```python
from build123d import *

# Parameters (mm, degrees)
F2_W     = 3.429
F2_H     = 3.429
F3_DEPTH = 25.4
F4_R     = 1.26999
F5_R     = 1.26999


# Not quite as in the source:
# - a fillet or chamfer is up to 0.001 mm smaller than in the source, because OpenCascade refuses the exact size


with BuildPart() as f1:
    # F0 (on Front) → F1 (revolve)
    with BuildSketch(Plane.XZ):
        Polygon((-1.27, 0), (0, 0), (4.445, 0), (4.445, 10.16), (0, 10.16), (-1.27, 10.16), (-1.27, 8.89), (0, 8.89), (0, 1.27), (-1.27, 1.27), align=None)
    revolve(axis=Axis((4.445, 0, 5.08), (0, 0, -1)))

    # F2 (on face) → F3 (cut)
    with BuildSketch(Plane(origin=(0, 0, 0), x_dir=(1, 0, 0), z_dir=(0, 0, -1))):
        with Locations((4.445, 0)):
            Rectangle(F2_W, F2_H)
    extrude(amount=-F3_DEPTH, mode=Mode.SUBTRACT)

    # F4 (radius 1.27 in the source; OpenCascade refuses exactly that, so slightly less here)
    f4_edges = [f1.edges().sort_by_distance(p)[0] for p in [
        (10.16, 0, 0),
    ]]
    fillet(f4_edges, radius=F4_R)

    # F5 (radius 1.27 in the source; OpenCascade refuses exactly that, so slightly less here)
    f5_edges = [f1.edges().sort_by_distance(p)[0] for p in [
        (10.16, 0, 10.16),
    ]]
    fillet(f5_edges, radius=F5_R)


solid = f1.part
```
Work out the finished part from the listing and answer in its coordinate system (mm). A direction names the side the tool comes from. Give positions to 0.01 mm unless a question says otherwise; leave off trailing zeros. Order: outer loops, then holes, each group sorted by start corner. A loop starts at its lowest first (then second) coordinate and runs counter-clockwise, first axis right, second up. Notation, with made-up numbers: (-27, -11) -> (-18, -11) arc R24 cw to (-18, 18) -> close; hole circle Ø3 at (8, 54). An arc over 180 degrees is marked (long way). Answer as CSV lines item,"result". Start each with the question number.
(1) For a pull along Z with two mould halves and no side action, classify faces 1 (the flat face through (8, -3, 8.89)), 2 (the flat face through (6.4, 0.1, 10.16)), 3 (the flat face through (4, -1.714, 5)) as released by +Z, released by -Z, zero draft, split by the parting line, or undercut.
(2) Each of these flat-tipped pins is pushed along its axis until it touches: pin 1 Ø1.7 at (y, z) = (0, 6.5) entering from +X; pin 2 Ø1.7 at (y, z) = (-0.5, 7) entering from -X; pin 3 Ø1 at (x, z) = (5, 2.5) entering from +Y. Where does it stop, or does it pass through?
(3) Section C-C, the plane z = 9.25 is taken. Write down the section's boundary in (x, y) (1 decimal).
(4) Consider line 1 along Y through (x, z) = (4.25, 7.75); line 2 along X through (y, z) = (0.5, 5); line 3 along Y through (x, z) = (4.25, 9). Determine where each line is inside the solid, lowest interval first.
(5) Which of the six approach directions +Z, -Z, +X, -X, +Y, -Y give full straight-line access (tool end or side, diameter ignored) to faces 4 (the cylindrical face through (5.41, -4.34, 5.03)), 5 (the flat face through (2.5, 0.1, 0)), 6 (the flat face through (6.16, 0, 5))?
(6) Section B-B, the plane z = 2.5 is taken. Write down the section's boundary in (x, y) (1 decimal), plus the area to 3 significant figures.
Entries:
1,face 1,"undercut"
1,face 2,"released by +Z"
1,face 3,"zero draft"
2,pin 1,"x = 8.89"
2,pin 2,"x = 0"
2,pin 3,"y = 4.44"
3,outline,"circle Ø11.3 at (4.4, 0); hole (2.7, -1.7) -> (6.2, -1.7) -> (6.2, 1.7) -> (2.7, 1.7) -> close"
4,line 1,"-4.44 to -1.71, 1.71 to 4.44"
4,line 2,"0.03 to 2.73, 6.16 to 8.86"
4,line 3,"-5.71 to -1.71, 1.71 to 5.71"
5,face 4,"none"
5,face 5,"-Z, +X, -X, +Y, -Y"
5,face 6,"+Z, -Z"
6,outline,"circle Ø8.9 at (4.4, 0); hole (2.7, -1.7) -> (6.2, -1.7) -> (6.2, 1.7) -> (2.7, 1.7) -> close"
6,area,"50.3 mm²"
